Build history of the part. All positions in model axes, mm. Give positions to 0.01 mm unless a question says otherwise; leave off trailing zeros. Answer as a JSON object with one key per item and string values. Group by question number.
1. Mould opens along Y. For faces 1 (the face through (-12.7, 6, 2)), 2 (the face through (0, 0, 2)) say: released by +Y, released by -Y, zero draft, split by the parting line, or undercut.
2. Slice it at A-A (z = 55.5). Give the number of separate pieces and of enclosed holes in the cut face, then the cut area to 3 significant figures.
3. Drill centre lines: line 1 along X through (y, z) = (4.75, -63); line 2 along Y through (x, z) = (6, 3.5); line 3 along Y through (x, z) = (-8.75, 161). Where is each one in solid material? Low to high. Write a range as [from, to].
4. Drop flat-ended pins along their axis: pin 1 Ø2.5 at (x, y) = (8.73, 3.96) entering from -Z; pin 2 Ø1.1 at (x, z) = (-5.5, 39) entering from -Y; pin 3 Ø1.6 at (x, z) = (-0.5, 27.5) entering from +Y. Give the stop position or say it passes through.
from build123d import *

# Parameters (mm, degrees)
SKETCH1_R           = 2.032
BOSS_EXTRUDE1_DEPTH = 177.8


with BuildPart() as part:
    # Sketch1 → Boss-Extrude1 (new, symmetric)
    with BuildSketch(Plane.XY):
        with BuildLine():
            Line((-12.7, 10.591838253), (-12.7, 2.108161747))
            ThreePointArc((-12.7, 2.108161747), (-12.078025605, 0.612955845), (-10.5791, 0))
            ThreePointArc((-10.5791, 0), (-10.06475, 0.508039196), (-9.5504, 0))
            Line((-9.5504, 0), (-6.3246, 0))
            ThreePointArc((-6.3246, 0), (-5.8166, 0.508), (-5.3086, 0))
            Line((-5.3086, 0), (5.3086, 0))
            ThreePointArc((5.3086, 0), (5.8166, 0.508), (6.3246, 0))
            Line((6.3246, 0), (9.5504, 0))
            ThreePointArc((9.5504, 0), (10.06475, 0.508039196), (10.5791, 0))
            ThreePointArc((10.5791, 0), (12.078025605, 0.612955845), (12.7, 2.108161747))
            Line((12.7, 2.108161747), (12.7, 10.591838253))
            ThreePointArc((12.7, 10.591838253), (12.078025605, 12.087044155), (10.5791, 12.7))
            ThreePointArc((10.5791, 12.7), (10.06475, 12.191960804), (9.5504, 12.7))
            Line((9.5504, 12.7), (6.3246, 12.7))
            ThreePointArc((6.3246, 12.7), (5.816599999, 12.191999983), (5.3086, 12.700000002))
            Line((5.3086, 12.700000002), (4.302307889, 12.700000002))
            ThreePointArc((4.302307889, 12.700000002), (3.197407889, 11.595100002), (4.302307889, 10.490200002))
            Line((4.302307889, 10.490200002), (6.487959021, 10.490200002))
            ThreePointArc((6.487959021, 10.490200002), (7.426620626, 9.863006369), (7.20637951, 8.755779512))
            Line((7.20637951, 8.755779512), (3.87633597, 5.425735971))
            ThreePointArc((3.87633597, 5.425735971), (2.846291837, 4.737482486), (1.631271939, 4.495800002))
            Line((1.631271939, 4.495800002), (-1.631271939, 4.495800002))
            ThreePointArc((-1.631271939, 4.495800002), (-2.846291837, 4.737482486), (-3.87633597, 5.425735971))
            Line((-3.87633597, 5.425735971), (-7.20637951, 8.755779512))
            ThreePointArc((-7.20637951, 8.755779512), (-7.426620626, 9.863006369), (-6.487959021, 10.490200002))
            Line((-6.487959021, 10.490200002), (-4.302307889, 10.490200002))
            ThreePointArc((-4.302307889, 10.490200002), (-3.197407889, 11.595100002), (-4.302307889, 12.700000002))
            Line((-4.302307889, 12.700000002), (-5.3086, 12.700000002))
            ThreePointArc((-5.3086, 12.700000002), (-5.816599999, 12.191999985), (-6.3246, 12.7))
            Line((-6.3246, 12.7), (-9.5504, 12.7))
            ThreePointArc((-9.5504, 12.7), (-10.06475, 12.191960804), (-10.5791, 12.7))
            ThreePointArc((-10.5791, 12.7), (-12.078025605, 12.087044155), (-12.7, 10.591838253))
        make_face()
        with Locations((-8.73125, 3.9624)):
            Circle(SKETCH1_R, mode=Mode.SUBTRACT)
        with Locations((8.73125, 3.9624)):
            Circle(SKETCH1_R, mode=Mode.SUBTRACT)
    extrude(amount=BOSS_EXTRUDE1_DEPTH, both=True)


solid = part.part
Established:
{
 "1": {"face 1": "zero draft", "face 2": "released by -Y"},
 "2": {"separate pieces": "1", "enclosed holes": "2", "area": "206 mm^2"},
 "3": {"line 1": "x = [-12.7, -10.6], [-6.86, -2.88], [2.88, 6.86], [10.6, 12.7]", "line 2": "y = [0.47, 7.55], [10.49, 12.23]", "line 3": "y = [0, 1.93], [5.99, 12.7]"},
 "4": {"pin 1": "passes through", "pin 2": "stops at y = 0", "pin 3": "stops at y = 4.5"}
}
